from build123d import *

# Parameters (mm, degrees)
SKETCH2_R           = 18
BOSS_EXTRUDE1_DEPTH = 1.3
BOSS_EXTRUDE7_START = -1.3
BOSS_EXTRUDE7_DEPTH = 1.3
SKETCH17_R          = 0.7
BOSS_EXTRUDE9_DEPTH = 1.3
BOSS_EXTRUDE2_START = -1.3
SKETCH3_R           = 35
SKETCH3_R_2         = 18
BOSS_EXTRUDE2_DEPTH = 1.3
SKETCH6_R           = 5
BOSS_EXTRUDE4_DEPTH = 1
SKETCH7_R           = 59.131365533
CUT_EXTRUDE1_DEPTH  = 10
FILLET1_R           = 6
SKETCH4_R           = 3.2
CUT_EXTRUDE2_DEPTH  = 10
SKETCH18_R          = 18
CUT_EXTRUDE3_DEPTH  = 10


with BuildPart() as part:
    # Sketch2 → Boss-Extrude1 (new body)
    with BuildSketch(Plane.XY.offset(10)):
        Circle(SKETCH2_R)
        with BuildLine():
            ThreePointArc((0, 0.538550206), (0.166421166, 0.512191682), (0.316551869, 0.435696269))
            Line((0.316551869, 0.435696269), (9.992349289, 13.753288904))
            ThreePointArc((9.992349289, 13.753288904), (13.753288904, 9.992349289), (16.167960777, 5.253288904))
            Line((16.167960777, 5.253288904), (0.512191682, 0.166421166))
            ThreePointArc((0.512191682, 0.166421166), (0.538550206, 0), (0.512191682, -0.166421166))
            Line((0.512191682, -0.166421166), (16.167960777, -5.253288904))
            ThreePointArc((16.167960777, -5.253288904), (13.753288904, -9.992349289), (9.992349289, -13.753288904))
            Line((9.992349289, -13.753288904), (0.316551869, -0.435696269))
            ThreePointArc((0.316551869, -0.435696269), (0.166421166, -0.512191682), (0, -0.538550206))
            Line((0, -0.538550206), (0, -17))
            ThreePointArc((0, -17), (-5.253288904, -16.167960777), (-9.992349289, -13.753288904))
            Line((-9.992349289, -13.753288904), (-0.316551869, -0.435696269))
            ThreePointArc((-0.316551869, -0.435696269), (-0.435696269, -0.316551869), (-0.512191682, -0.166421166))
            Line((-0.512191682, -0.166421166), (-16.167960777, -5.253288904))
            ThreePointArc((-16.167960777, -5.253288904), (-17, 0), (-16.167960777, 5.253288904))
            Line((-16.167960777, 5.253288904), (-0.512191682, 0.166421166))
            ThreePointArc((-0.512191682, 0.166421166), (-0.435696269, 0.316551869), (-0.316551869, 0.435696269))
            Line((-0.316551869, 0.435696269), (-9.992349289, 13.753288904))
            ThreePointArc((-9.992349289, 13.753288904), (-5.253288904, 16.167960777), (0, 17))
            Line((0, 17), (0, 0.538550206))
        make_face(mode=Mode.SUBTRACT)
        with BuildLine():
            Line((0.5, 1.198581445), (0.5, 16.492422502))
            ThreePointArc((0.5, 16.492422502), (5.193820321, 15.661233364), (9.454148381, 13.522909391))
            Line((9.454148381, 13.522909391), (0.5, 1.198581445))
        make_face(mode=Mode.SUBTRACT)
        with BuildLine():
            Line((-9.939558578, 13.170238239), (-0.985410197, 0.845910294))
            Line((-0.985410197, 0.845910294), (-15.530717393, 5.57196709))
            ThreePointArc((-15.530717393, 5.57196709), (-13.289739299, 9.779203923), (-9.939558578, 13.170238239))
        make_face(mode=Mode.SUBTRACT)
        with BuildLine():
            Line((-15.597133416, -5.383254519), (-1.109016994, -0.675780132))
            Line((-1.109016994, -0.675780132), (-10.098511219, -13.048757457))
            ThreePointArc((-10.098511219, -13.048757457), (-13.40733091, -9.617352956), (-15.597133416, -5.383254519))
        make_face(mode=Mode.SUBTRACT)
        with BuildLine():
            ThreePointArc((9.289494224, -13.636542709), (5.003553098, -15.723054932), (0.3, -16.497272502))
            Line((0.3, -16.497272502), (0.3, -1.263565384))
            Line((0.3, -1.263565384), (9.289494224, -13.636542709))
        make_face(mode=Mode.SUBTRACT)
        with BuildLine():
            Line((15.782543612, -4.812620609), (1.294427191, -0.105146222))
            Line((1.294427191, -0.105146222), (15.839734388, 4.620910574))
            ThreePointArc((15.839734388, 4.620910574), (16.499696789, -0.100029399), (15.782543612, -4.812620609))
        make_face(mode=Mode.SUBTRACT)
    extrude(amount=-BOSS_EXTRUDE1_DEPTH)

    # Sketch11 → Boss-Extrude7 (add)
    with BuildSketch(Plane(origin=(0, 0, 8.7), x_dir=(-1, 0, 0), z_dir=(0, 0, -1)).offset(BOSS_EXTRUDE7_START)):
        with BuildLine():
            ThreePointArc((-0.512191682, 0.166421166), (-0.435696269, 0.316551869), (-0.316551869, 0.435696269))
            Line((-0.316551869, 0.435696269), (-9.992349289, 13.753288904))
            ThreePointArc((-9.992349289, 13.753288904), (-13.753288904, 9.992349289), (-16.167960777, 5.253288904))
            Line((-16.167960777, 5.253288904), (-0.512191682, 0.166421166))
        make_face()
        with BuildLine():
            Line((0, 17), (0, 0.538550206))
            ThreePointArc((0, 0.538550206), (0.166421166, 0.512191682), (0.316551869, 0.435696269))
            Line((0.316551869, 0.435696269), (9.992349289, 13.753288904))
            ThreePointArc((9.992349289, 13.753288904), (5.253288904, 16.167960777), (0, 17))
        make_face()
        with BuildLine():
            Line((16.167960777, 5.253288904), (0.512191682, 0.166421166))
            ThreePointArc((0.512191682, 0.166421166), (0.531919759, 0.084247813), (0.538550206, 0))
            ThreePointArc((0.538550206, 0), (0.531919759, -0.084247813), (0.512191682, -0.166421166))
            Line((0.512191682, -0.166421166), (16.167960777, -5.253288904))
            ThreePointArc((16.167960777, -5.253288904), (17, 0), (16.167960777, 5.253288904))
        make_face()
        with BuildLine():
            Line((9.992349289, -13.753288904), (0.316551869, -0.435696269))
            ThreePointArc((0.316551869, -0.435696269), (0.166421166, -0.512191682), (0, -0.538550206))
            Line((0, -0.538550206), (0, -17))
            ThreePointArc((0, -17), (5.253288904, -16.167960777), (9.992349289, -13.753288904))
        make_face()
        with BuildLine():
            ThreePointArc((-0.316551869, -0.435696269), (-0.435696269, -0.316551869), (-0.512191682, -0.166421166))
            Line((-0.512191682, -0.166421166), (-16.167960777, -5.253288904))
            ThreePointArc((-16.167960777, -5.253288904), (-13.753288904, -9.992349289), (-9.992349289, -13.753288904))
            Line((-9.992349289, -13.753288904), (-0.316551869, -0.435696269))
        make_face()
        with BuildLine():
            ThreePointArc((0.316551869, 0.435696269), (0.166421166, 0.512191682), (0, 0.538550206))
            ThreePointArc((0, 0.538550206), (-0.166421166, 0.512191682), (-0.316551869, 0.435696269))
            ThreePointArc((-0.316551869, 0.435696269), (-0.435696269, 0.316551869), (-0.512191682, 0.166421166))
            ThreePointArc((-0.512191682, 0.166421166), (-0.538550206, 0), (-0.512191682, -0.166421166))
            ThreePointArc((-0.512191682, -0.166421166), (-0.435696269, -0.316551869), (-0.316551869, -0.435696269))
            ThreePointArc((-0.316551869, -0.435696269), (-0.166421166, -0.512191682), (0, -0.538550206))
            ThreePointArc((0, -0.538550206), (0.166421166, -0.512191682), (0.316551869, -0.435696269))
            ThreePointArc((0.316551869, -0.435696269), (0.435696269, -0.316551869), (0.512191682, -0.166421166))
            ThreePointArc((0.512191682, -0.166421166), (0.531919759, -0.084247813), (0.538550206, 0))
            ThreePointArc((0.538550206, 0), (0.531919759, 0.084247813), (0.512191682, 0.166421166))
            ThreePointArc((0.512191682, 0.166421166), (0.435696269, 0.316551869), (0.316551869, 0.435696269))
        make_face()
    extrude(amount=BOSS_EXTRUDE7_DEPTH)

    # Sketch17 → Boss-Extrude9 (add)
    with BuildSketch(Plane(origin=(0, 0, 8.7), x_dir=(-1, 0, 0), z_dir=(0, 0, -1))):
        Circle(SKETCH17_R)
    extrude(amount=-BOSS_EXTRUDE9_DEPTH)

    # Sketch3 → Boss-Extrude2 (add)
    with BuildSketch(Plane(origin=(0, 0, 8.7), x_dir=(-1, 0, 0), z_dir=(0, 0, -1)).offset(BOSS_EXTRUDE2_START)):
        Circle(SKETCH3_R)
        Circle(SKETCH3_R_2, mode=Mode.SUBTRACT)
    extrude(amount=BOSS_EXTRUDE2_DEPTH)

    # Sketch6 → Boss-Extrude4 (add)
    with BuildSketch(Plane(origin=(0, 0, 10), x_dir=(-1, 0, 0), z_dir=(0, 0, -1))):
        with Locations((0, 30)):
            Circle(SKETCH6_R)
        with Locations((25.980762114, -15)):
            Circle(SKETCH6_R)
        with Locations((-25.980762114, -15)):
            Circle(SKETCH6_R)
    extrude(amount=BOSS_EXTRUDE4_DEPTH)

    # Sketch7 → Cut-Extrude1 (cut)
    with BuildSketch(Plane(origin=(0, 0, 8.7), x_dir=(-1, 0, 0), z_dir=(0, 0, -1))):
        Circle(SKETCH7_R)
        Polygon((0, 42), (-36.373066959, -21), (36.373066959, -21), align=None, mode=Mode.SUBTRACT)
    extrude(amount=-CUT_EXTRUDE1_DEPTH, mode=Mode.SUBTRACT)

    # Fillet1
    fillet1_edges = [part.edges().sort_by_distance(p)[0] for p in [
        (4.186533479, 34.748711306, 9.35),
        (32.186533479, -13.748711306, 9.35),
        (28, -21, 9.35),
        (-28, -21, 9.35),
        (-32.186533479, -13.748711306, 9.35),
        (-4.186533479, 34.748711306, 9.35),
    ]]
    fillet(fillet1_edges, radius=FILLET1_R)

    # Sketch4 → Cut-Extrude2 (cut)
    with BuildSketch(Plane(origin=(0, 0, 8.7), x_dir=(-1, 0, 0), z_dir=(0, 0, -1))):
        with Locations((0, 29)):
            Circle(SKETCH4_R)
        with Locations((25.11473671, -14.5)):
            Circle(SKETCH4_R)
        with Locations((-25.11473671, -14.5)):
            Circle(SKETCH4_R)
    extrude(amount=-CUT_EXTRUDE2_DEPTH, mode=Mode.SUBTRACT)

    # Sketch18 → Cut-Extrude3 (cut)
    with BuildSketch(Plane.XY.offset(10)):
        Circle(SKETCH18_R)
    extrude(amount=-CUT_EXTRUDE3_DEPTH, mode=Mode.SUBTRACT)


solid = part.part
For this review, take the finished solid that the model builds, in its own axes (mm). Coordinates: 2 decimals unless noted, no trailing zeros. Loops run counter-clockwise (first coordinate to the right, second up) from the corner with the lowest first, then second, coordinate; pieces in that order, holes last. Notation, with made-up numbers: (20, 67) - (70, 67) arc R28 ccw to (70, 90) - close; hole circle Ø5 at (-0.5, -19). An arc over 180 degrees is marked (long way). Return JSON: item names as keys, results as strings.
Item 1: Take a section at A-A (x = 0). Give the boundary of the cut face in (y, z).
Determined:
{"outline": "(-21, 8.7) - (-18, 8.7) - (-18, 10) - (-21, 10) - close; (18, 8.7) - (25.8, 8.7) - (25.8, 10) - (18, 10) - close; (32.2, 8.7) - (35, 8.7) - (35, 10) - (32.2, 10) - close"}
Item 2: Take a section at D-D (y = -14.5). Give the boundary of the cut face in (x, z).
Determined:
{"outline": "(-31.38, 8.7) - (-28.31, 8.7) - (-28.31, 10) - (-31.38, 10) - close; (-21.91, 8.7) - (-10.67, 8.7) - (-10.67, 10) - (-21.91, 10) - close; (10.67, 8.7) - (21.91, 8.7) - (21.91, 10) - (10.67, 10) - close; (28.31, 8.7) - (31.38, 8.7) - (31.38, 10) - (28.31, 10) - close"}
Item 3: Insertion check: pin 1 (6 mm diameter, centred on x = 0, y = 29, fed in from +Z). The pin has a flat end and moves straight along its axis. Give the tip position at first contact, or say it passes through.
Determined:
{"pin 1": "passes through"}
Item 4: Mouldability with a two-part tool opening along X and no side actions: class faces 1 (the cylindrical face through (3.67, 34.14, 9.36)), 2 (the cylindrical face through (-2.343, 17.847, 9.359)), 3 (the flat face through (-18.36, 10.2, 9.34)) as pulls with the +X half, pulls with the -X half, needs draft (parallel to the pull), parting line crosses it, or undercut.
Determined:
{"face 1": "pulls with the +X half", "face 2": "undercut", "face 3": "pulls with the -X half"}
Item 5: Take a section at B-B (z = 9.45). Give the boundary of the cut face in (x, y).
Determined:
{"outline": "(-30.66, -16.89) arc R35 ccw to (-29.95, -18.1) arc R6 ccw to (-24.82, -21) - (24.82, -21) arc R6 ccw to (29.95, -18.1) arc R35 ccw to (30.66, -16.89) arc R6 ccw to (30.6, -10.99) - (5.78, 31.99) arc R6 ccw to (0.7, 34.99) arc R35 ccw to (-0.7, 34.99) arc R6 ccw to (-5.78, 31.99) - (-30.6, -10.99) arc R6 ccw to start; hole circle Ø6.4 at (-25.11, -14.5); hole circle Ø36 at (0, 0); hole circle Ø6.4 at (0, 29); hole circle Ø6.4 at (25.11, -14.5)"}
Item 6: For line 1 (Y direction, x = 0, z = 9.55); line 2 (Y direction, x = 2.5, z = 8.8); line 3 (Y direction, x = -24, z = 8.85), list the stretches that pass through material, from the lowest coordinate up.
Determined:
{"line 1": "y = -21 to -18, 18 to 25.8, 32.2 to 35", "line 2": "y = -21 to -17.83, 17.83 to 27, 31 to 34.68", "line 3": "y = -21 to -17.5, -11.5 to 0.43"}
Item 7: Take a section at C-C (y = 1.5). Give the boundary of the cut face in (x, z).
Determined:
{"outline": "(-23.38, 8.7) - (-17.94, 8.7) - (-17.94, 10) - (-23.38, 10) - close; (17.94, 8.7) - (23.38, 8.7) - (23.38, 10) - (17.94, 10) - close"}
